Design review of the part built by this model. Coordinates are the model's own, in mm. Give positions to 0.01 mm unless a question says otherwise; leave off trailing zeros. Loops run counter-clockwise (first coordinate to the right, second up) from the corner with the lowest first, then second, coordinate; pieces in that order, holes last. Notation, with made-up numbers: M 48,32.5 L 63,32.5 A23 ccw 63,49.5 Z; hole C 2,-33.5 d1. An arc over 180 degrees is marked long. Use a Markdown table: item, result. Add a question column.
(1) Add section D-D, the plane x = 8. Give the boundary of the cut face in (y, z), then the cut area to 3 significant figures.
(2) Insertion check: pin 1 Ø2 at (x, z) = (-9, 4) entering from -Y; pin 2 Ø3 at (x, z) = (9, 3) entering from +Y; pin 3 Ø4 at (x, z) = (-13.5, 5.5) entering from +Y. Each pin has a flat end and moves straight along its axis. Give the tip position at first contact, or say it passes through.
(3) Add section A-A, the plane z = 5.25. Give the boundary of the cut face in (x, y), then the cut area to 3 significant figures.
(4) For probe 1 along Y at (x, z) = (-11.5, 2.5); probe 2 along X at (y, z) = (-7, 6); probe 3 along X at (y, z) = (-5.5, 2), list the stretches that pass through material, from the lowest coordinate up.
(5) Add section B-B, the plane x = 0. Give the boundary of the cut face in (y, z), then the cut area to 3 significant figures.
(6) Add section C-C, the plane y = 0. Give the boundary of the cut face in (x, z).
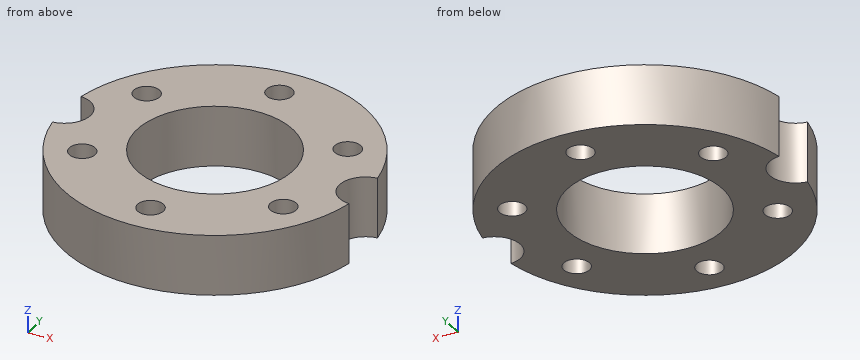
```python
from build123d import *

# Parameters (mm, degrees)
SKETCH_1_R      = 1.5
SKETCH_1_R_2    = 9
EXTRUDE_1_DEPTH = 7


with BuildPart() as part:
    # 草图1 → 凸台-拉伸1 (new body)
    with BuildSketch(Plane.XY):
        with BuildLine():
            ThreePointArc((17.242857143, -2.988959276), (14.5, 0), (17.242857143, 2.988959276))
            ThreePointArc((17.242857143, 2.988959276), (0, 17.5), (-17.242857143, 2.988959276))
            ThreePointArc((-17.242857143, 2.988959276), (-14.5, 0), (-17.242857143, -2.988959276))
            ThreePointArc((-17.242857143, -2.988959276), (0, -17.5), (17.242857143, -2.988959276))
        make_face()
        with Locations((-11.691342951, -6.75)):
            Circle(SKETCH_1_R, mode=Mode.SUBTRACT)
        with Locations((0, -13.5)):
            Circle(SKETCH_1_R, mode=Mode.SUBTRACT)
        with Locations((11.691342951, -6.75)):
            Circle(SKETCH_1_R, mode=Mode.SUBTRACT)
        with Locations((-11.691342951, 6.75)):
            Circle(SKETCH_1_R, mode=Mode.SUBTRACT)
        Circle(SKETCH_1_R_2, mode=Mode.SUBTRACT)
        with Locations((11.691342951, 6.75)):
            Circle(SKETCH_1_R, mode=Mode.SUBTRACT)
        with Locations((0, 13.5)):
            Circle(SKETCH_1_R, mode=Mode.SUBTRACT)
    extrude(amount=EXTRUDE_1_DEPTH)


solid = part.part
```
Established:
| question | item | result |
|---|---|---|
| 1 | outline | M -15.56,0 L -4.12,0 L -4.12,7 L -15.56,7 Z; M 4.12,0 L 15.56,0 L 15.56,7 L 4.12,7 Z |
| 1 | area | 160 mm^2 |
| 2 | pin 1 | y = -15.56 |
| 2 | pin 2 | y = 15.81 |
| 2 | pin 3 | y = 13.19 |
| 3 | outline | M -17.24,-2.99 A17.5 ccw 17.24,-2.99 A3 cw 17.24,2.99 A17.5 ccw -17.24,2.99 A3 cw Z; hole C -11.69,-6.75 d3; hole C -11.69,6.75 d3; hole C 0,0 d18; hole C 0,-13.5 d3; hole C 0,13.5 d3; hole C 11.69,-6.75 d3; hole C 11.69,6.75 d3 |
| 3 | area | 638 mm^2 |
| 4 | probe 1 | -13.19 to -8.24, -5.26 to 5.26, 8.24 to 13.19 |
| 4 | probe 2 | -16.04 to -13.17, -10.21 to -5.66, 5.66 to 10.21, 13.17 to 16.04 |
| 4 | probe 3 | -16.61 to -12.52, -10.86 to -7.12, 7.12 to 10.86, 12.52 to 16.61 |
| 5 | outline | M -17.5,0 L -15,0 L -15,7 L -17.5,7 Z; M -12,0 L -9,0 L -9,7 L -12,7 Z; M 9,0 L 12,0 L 12,7 L 9,7 Z; M 15,0 L 17.5,0 L 17.5,7 L 15,7 Z |
| 5 | area | 77.0 mm^2 |
| 6 | outline | M -14.5,0 L -9,0 L -9,7 L -14.5,7 Z; M 9,0 L 14.5,0 L 14.5,7 L 9,7 Z |
